For this review, take the finished solid that the model builds, in its own axes (mm). Face numbers are marked on the shaded views. Coordinates: 2 decimals unless noted, no trailing zeros. Write each loop counter-clockwise with the first axis right and the second up, starting at its lowest first coordinate (ties: lowest second). Pieces come first, ordered by that corner, then holes. Notation, with made-up numbers: M 28,53.5 L 57,53.5 A28 cw 57,78.5 Z; hole C -19,0 d7. An arc over 180 degrees is marked long. Return JSON: item names as keys, results as strings.
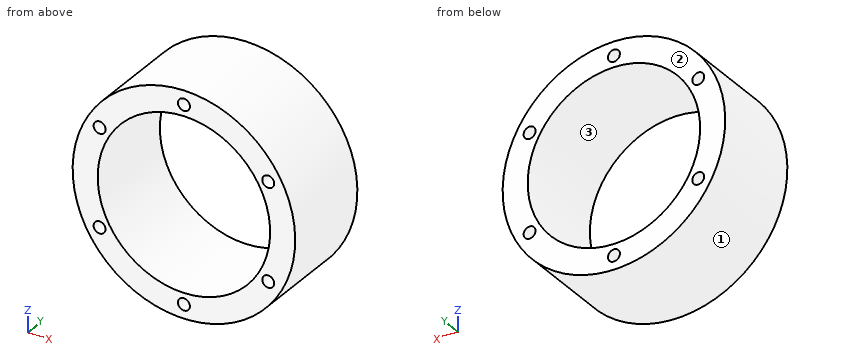
```python
from build123d import *

# Parameters (mm, degrees)
SKETCH_1_R      = 40
SKETCH_1_R_2    = 31
SKETCH_1_R_3    = 2.15
EXTRUDE_3_DEPTH = 15
SKETCH_2_R      = 40
SKETCH_2_R_2    = 31
SKETCH_2_R_3    = 2.15
EXTRUDE_5_DEPTH = 20


with BuildPart() as part:
    # 草图1 → 凸台-拉伸3 (new body)
    with BuildSketch(Plane(origin=(0, 0, 0), x_dir=(1, 0, 0), z_dir=(0, 1, 0))):
        with Locations(Location((0, 0, 0), (0, 0, 270))):
            Circle(SKETCH_1_R)
        with Locations(Location((0, 0, 0), (0, 0, 270))):
            Circle(SKETCH_1_R_2, mode=Mode.SUBTRACT)
        with Locations(Location((0, 35, 0), (0, 0, 270))):
            Circle(SKETCH_1_R_3, mode=Mode.SUBTRACT)
        with Locations(Location((30.310889132, 17.5, 0), (0, 0, 270))):
            Circle(SKETCH_1_R_3, mode=Mode.SUBTRACT)
        with Locations(Location((30.310889132, -17.5, 0), (0, 0, 270))):
            Circle(SKETCH_1_R_3, mode=Mode.SUBTRACT)
        with Locations(Location((0, -35, 0), (0, 0, 270))):
            Circle(SKETCH_1_R_3, mode=Mode.SUBTRACT)
        with Locations(Location((-30.310889132, -17.5, 0), (0, 0, 270))):
            Circle(SKETCH_1_R_3, mode=Mode.SUBTRACT)
        with Locations(Location((-30.310889132, 17.5, 0), (0, 0, 270))):
            Circle(SKETCH_1_R_3, mode=Mode.SUBTRACT)
    extrude(amount=EXTRUDE_3_DEPTH)

    # 草图2 → 凸台-拉伸5 (add)
    with BuildSketch(Plane(origin=(0, 15, 0), x_dir=(1, 0, 0), z_dir=(0, 1, 0))):
        with Locations(Location((0, 0, 0), (0, 0, 270))):
            Circle(SKETCH_2_R)
        with Locations(Location((0, 0, 0), (0, 0, 270))):
            Circle(SKETCH_2_R_2, mode=Mode.SUBTRACT)
        with Locations(Location((0, 35, 0), (0, 0, 270))):
            Circle(SKETCH_2_R_3, mode=Mode.SUBTRACT)
        with Locations(Location((30.310889132, 17.5, 0), (0, 0, 270))):
            Circle(SKETCH_2_R_3, mode=Mode.SUBTRACT)
        with Locations(Location((30.310889132, -17.5, 0), (0, 0, 270))):
            Circle(SKETCH_2_R_3, mode=Mode.SUBTRACT)
        with Locations(Location((0, -35, 0), (0, 0, 270))):
            Circle(SKETCH_2_R_3, mode=Mode.SUBTRACT)
        with Locations(Location((-30.310889132, -17.5, 0), (0, 0, 270))):
            Circle(SKETCH_2_R_3, mode=Mode.SUBTRACT)
        with Locations(Location((-30.310889132, 17.5, 0), (0, 0, 270))):
            Circle(SKETCH_2_R_3, mode=Mode.SUBTRACT)
    extrude(amount=EXTRUDE_5_DEPTH)


solid = part.part
```
1. Clearance check with flat-ended pins moving along their axes: pin 1 Ø2.5 at (x, z) = (30.31, 17.5) entering from +Y; pin 2 Ø1.5 at (x, y) = (-29, 22.5) entering from -Z; pin 3 Ø2 at (y, z) = (20.5, -20) entering from -X; pin 4 Ø4 at (y, z) = (7, 24.5) entering from +X. State where each tip first meets the part, or that it passes through.
Checks:
{"pin 1": "through", "pin 2": "z = -28.32", "pin 3": "x = -35.2", "pin 4": "x = 33.07"}
2. Wall thickness on L1, parallel to X at y = 16, z = -17; L2, parallel to X at y = 13.5, z = 0; L3, parallel to X at y = 17.5, z = -19: over which ranges is each line inside the solid? List them lowest first. Write a range as from..to.
Checks:
{"L1": "-36.21..-32.4, -28.22..-25.92, 25.92..28.22, 32.4..36.21", "L2": "-40..-31, 31..40", "L3": "-35.2..-31.85, -28.77..-24.49, 24.49..28.77, 31.85..35.2"}
3. We need section B-B (z = 0). State the section outline as (x, y) points.
Checks:
{"outline": "M -40,0 L -31,0 L -31,35 L -40,35 Z; M 31,0 L 40,0 L 40,35 L 31,35 Z"}
4. Draft analysis for pull direction Z (two halves, no side actions). For the marked faces 1, 2 and 3, state which applies: +Z half, -Z half, draft (parallel to the pull), parting line (faces both ways), or undercut.
Checks:
{"face 1": "parting line", "face 2": "draft", "face 3": "undercut"}
5. We need section C-C (y = 11). State the section outline as (x, z) points.
Checks:
{"outline": "C 0,0 d80; hole C -30.31,-17.5 d4.3; hole C -30.31,17.5 d4.3; hole C 0,0 d62; hole C 0,-35 d4.3; hole C 0,35 d4.3; hole C 30.31,-17.5 d4.3; hole C 30.31,17.5 d4.3"}
6. We need section A-A (x = 0). State the section outline as (y, z) points, plus the area to 3 significant figures.
Checks:
{"outline": "M 0,-40 L 35,-40 L 35,-37.15 L 0,-37.15 Z; M 0,-32.85 L 35,-32.85 L 35,-31 L 0,-31 Z; M 0,31 L 35,31 L 35,32.85 L 0,32.85 Z; M 0,37.15 L 35,37.15 L 35,40 L 0,40 Z", "area": "329 mm2"}
7. We need section D-D (z = 17.5). State the section outline as (x, y) points.
Checks:
{"outline": "M -35.97,0 L -32.46,0 L -32.46,35 L -35.97,35 Z; M -28.16,0 L -25.59,0 L -25.59,35 L -28.16,35 Z; M 25.59,0 L 28.16,0 L 28.16,35 L 25.59,35 Z; M 32.46,0 L 35.97,0 L 35.97,35 L 32.46,35 Z"}
